Verification items for the finished model (mm, model axes). Face numbers are marked on the shaded views. Give positions to 0.01 mm unless a question says otherwise; leave off trailing zeros. Write each loop counter-clockwise with the first axis right and the second up, starting at its lowest first coordinate (ties: lowest second). Pieces come first, ordered by that corner, then holes.
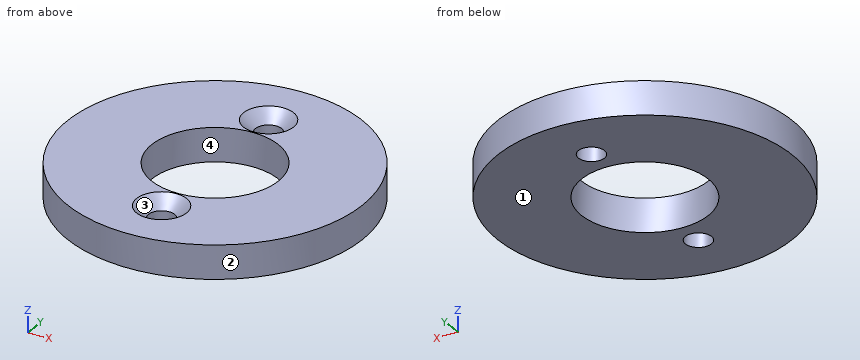
from build123d import *

# Parameters (mm, degrees)
SKETCH_1_R                    = 39.5
EXTRUDE_1_DEPTH               = 9
CUT_EXTRUDE_1_DEPTH           = 57.581799194
CUT_EXTRUDE_1_DEPTH_BACK      = 57.581799194
SKETCH_2_R                    = 17
SKETCH_2_R_2                  = 3.5
SKETCH_3_R                    = 6.72
CUT_EXTRUDE_2_DEPTH           = 3.22
CUT_EXTRUDE_2_DRAFT           = -45
CUT_EXTRUDE_2_PROFILE_2_DEPTH = 3.22
CUT_EXTRUDE_2_PROFILE_2_DRAFT = -45


with BuildPart() as part:
    # ｽｹｯﾁ1 → ﾎﾞｽ - 押し出し1 (new body)
    with BuildSketch(Plane.XY):
        Circle(SKETCH_1_R)
    extrude(amount=EXTRUDE_1_DEPTH)

    # ｽｹｯﾁ2 → ｶｯﾄ - 押し出し1 (cut, two sides: drawn at the far end of the back side and taken through both)
    with BuildSketch(Plane.XY.offset(-CUT_EXTRUDE_1_DEPTH_BACK)):
        Circle(SKETCH_2_R)
        with Locations((0, 24)):
            Circle(SKETCH_2_R_2)
        with Locations((0, -24)):
            Circle(SKETCH_2_R_2)
    extrude(amount=CUT_EXTRUDE_1_DEPTH + CUT_EXTRUDE_1_DEPTH_BACK, mode=Mode.SUBTRACT)


with BuildPart() as cut_extrude_2_tool:
    # ｽｹｯﾁ3 → ｶｯﾄ - 押し出し2 (with draft: the straight prism first)
    with BuildSketch(Plane.XY.offset(9)):
        with Locations((0, 24)):
            Circle(SKETCH_3_R)
    extrude(amount=-CUT_EXTRUDE_2_DEPTH)
    # ｶｯﾄ - 押し出し2: the draft: its side faces are tilted about the plane it starts from
    cut_extrude_2_sides = [cut_extrude_2_tool.faces().sort_by_distance(p)[0] for p in [
        (-6.72, 24, 7.39),
    ]]
    draft(cut_extrude_2_sides, Plane.XY.offset(9), CUT_EXTRUDE_2_DRAFT)


with BuildPart() as part_1:
    add(part.part)

    # ｶｯﾄ - 押し出し2: cut by cut_extrude_2_tool
    add(cut_extrude_2_tool.part, mode=Mode.SUBTRACT)


with BuildPart() as cut_extrude_2_profile_2_tool:
    # ｽｹｯﾁ3 → ｶｯﾄ - 押し出し2 profile 2 (with draft: the straight prism first)
    with BuildSketch(Plane.XY.offset(9)):
        with Locations((0, -24)):
            Circle(SKETCH_3_R)
    extrude(amount=-CUT_EXTRUDE_2_PROFILE_2_DEPTH)
    # ｶｯﾄ - 押し出し2 profile 2: the draft: its side faces are tilted about the plane it starts from
    cut_extrude_2_profile_2_sides = [cut_extrude_2_profile_2_tool.faces().sort_by_distance(p)[0] for p in [
        (-6.72, -24, 7.39),
    ]]
    draft(cut_extrude_2_profile_2_sides, Plane.XY.offset(9), CUT_EXTRUDE_2_PROFILE_2_DRAFT)


with BuildPart() as part_2:
    add(part_1.part)

    # ｶｯﾄ - 押し出し2 profile 2: cut by cut_extrude_2_profile_2_tool
    add(cut_extrude_2_profile_2_tool.part, mode=Mode.SUBTRACT)


solid = part_2.part
Item 1: Scan lines: line 1 along Y through (x, z) = (0, 2.65); line 2 along Y through (x, z) = (0, 7); line 3 along X through (y, z) = (25.5, 6.25). Record each from-to range of solid material in increasing order.
Answer key:
line 1: y = -39.5 to -27.5, -20.5 to -17, 17 to 20.5, 27.5 to 39.5
line 2: y = -39.5 to -28.72, -19.28 to -17, 17 to 19.28, 28.72 to 39.5
line 3: x = -30.17 to -3.68, 3.68 to 30.17
Item 2: Release check for a two-part mould opening along X. For the marked faces 1, 2, 3 and 4 record: released by +X, released by -X, zero draft, split by the parting line, or undercut.
Answer key:
face 1: zero draft
face 2: split by the parting line
face 3: undercut
face 4: undercut
Item 3: Depth check by flat-ended pin: pin 1 (20.5 mm diameter, centred on x = 0, y = 0, fed in from -Z); pin 2 (2 mm diameter, centred on y = -9, z = 5.5, fed in from +X); pin 3 (3 mm diameter, centred on x = -17, z = 7, fed in from -Y); pin 4 (2 mm diameter, centred on y = -23.5, z = 4, fed in from +X). Enter the tip coordinate at first touch or a pass-through.
Answer key:
pin 1: passes through
pin 2: stops at x = 38.68
pin 3: stops at y = -36.33
pin 4: stops at x = 32.47
Item 4: Sectioned sample at A-A on y = 0. Record the cut outline in (x, z), then the cut area to 3 significant figures.
Answer key:
outline: (-39.5, 0) - (-17, 0) - (-17, 9) - (-39.5, 9) - close; (17, 0) - (39.5, 0) - (39.5, 9) - (17, 9) - close
area: 405 mm2
Item 5: Sectioned sample at C-C on z = 1.75. Record the cut outline in (x, y), then the cut area to 3 significant figures.
Answer key:
outline: circle Ø79 at (0, 0); hole circle Ø34 at (0, 0); hole circle Ø7 at (0, -24); hole circle Ø7 at (0, 24)
area: 3,920 mm2
Item 6: Sectioned sample at D-D on z = 7. Record the cut outline in (x, y).
Answer key:
outline: circle Ø79 at (0, 0); hole circle Ø34 at (0, 0); hole circle Ø9.44 at (0, -24); hole circle Ø9.44 at (0, 24)
Item 7: Sectioned sample at B-B on x = 0. Record the cut outline in (y, z), then the cut area to 3 significant figures.
Answer key:
outline: (-39.5, 0) - (-27.5, 0) - (-27.5, 5.78) - (-30.72, 9) - (-39.5, 9) - close; (-20.5, 0) - (-17, 0) - (-17, 9) - (-17.28, 9) - (-20.5, 5.78) - close; (17, 0) - (20.5, 0) - (20.5, 5.78) - (17.28, 9) - (17, 9) - close; (27.5, 0) - (39.5, 0) - (39.5, 9) - (30.72, 9) - (27.5, 5.78) - close
area: 258 mm2
